Design review of the part built by this model. Coordinates are the model's own, in mm. A direction names the side the tool comes from. Coordinates: 2 decimals unless noted, no trailing zeros. Write item = value, one per line.
```python
from build123d import *

# Parameters (mm, degrees)
F1_DEPTH = 10
F1_TAPER = 3
F3_DEPTH = 1.5


with BuildPart() as f1:
    # F0 (on Top) → F1 (new body)
    with BuildSketch(Plane.XY):
        with BuildLine():
            Line((-97, -97), (97, -97))
            Line((97, -97), (97, 87))
            ThreePointArc((97, 87), (94.0710678119, 94.0710678119), (87, 97))
            Line((87, 97), (-87, 97))
            ThreePointArc((-87, 97), (-94.0710678119, 94.0710678119), (-97, 87))
            Line((-97, 87), (-97, -97))
        make_face()
        with BuildLine():
            Line((95, 87), (95, -95))
            Line((95, -95), (-95, -95))
            Line((-95, -95), (-95, 87))
            ThreePointArc((-95, 87), (-92.6568542495, 92.6568542495), (-87, 95))
            Line((-87, 95), (87, 95))
            ThreePointArc((87, 95), (92.6568542495, 92.6568542495), (95, 87))
        make_face(mode=Mode.SUBTRACT)
    extrude(amount=F1_DEPTH, taper=F1_TAPER)

    # F2 (on face) → F3 (join)
    with BuildSketch(Plane(origin=(0, 0, 0), x_dir=(1, 0, 0), z_dir=(0, 0, -1))):
        with BuildLine():
            Line((97, -87), (97, 97))
            Line((97, 97), (-97, 97))
            Line((-97, 97), (-97, -87))
            ThreePointArc((-97, -87), (-94.0710678119, -94.0710678119), (-87, -97))
            Line((-87, -97), (87, -97))
            ThreePointArc((87, -97), (94.0710678119, -94.0710678119), (97, -87))
        make_face()
    extrude(amount=F3_DEPTH)


solid = f1.part
```
(1) For L1, parallel to Y at x = -47, z = 9.5; L2, parallel to Y at x = -18, z = 1; L3, parallel to Z at x = 2, y = -39.5, list the stretches that pass through material, from the lowest coordinate up.
Report:
L1 = -96.5 to -95.5, 95.5 to 96.5
L2 = -96.95 to -95.05, 95.05 to 96.95
L3 = -1.5 to 0
(2) For faces 1 (the conical face through (-93.807, 93.958, 5.07)), 2 (the conical face through (92.78, 92.91, 5.07)), list the 3-axis set-ups (+Z, -Z, +X, -X, +Y, -Y) from which the entire face can be reached by the end or side of a thin tool; tool diameter is ignored.
Report:
face_1 = +Z, -X, +Y
face_2 = +Z
(3) The part is to be moulded in two halves that separate along X. For faces 3 (the flat face through (-1, -1, 0)), 4 (the flat face through (-1, -1, -1.5)), 5 (the cylindrical face through (93.99, 94.15, -0.74)), say which applies: released by +X, released by -X, zero draft, split by the parting line, or undercut.
Report:
face_3 = undercut
face_4 = zero draft
face_5 = released by +X
(4) Insertion check: pin 1 (5 mm diameter, centred on x = 23, z = 3.5, fed in from +Y); pin 2 (4 mm diameter, centred on y = 20, z = 1, fed in from -X); pin 3 (3 mm diameter, centred on x = 43, y = -38, fed in from +Z); pin 4 (3 mm diameter, centred on x = 13, z = 6.5, fed in from -Y). Each pin has a flat end and moves straight along its axis. Give the tip position at first contact, or say it passes through.
Report:
pin_1 = 96.95
pin_2 = -97
pin_3 = 0
pin_4 = -96.74
